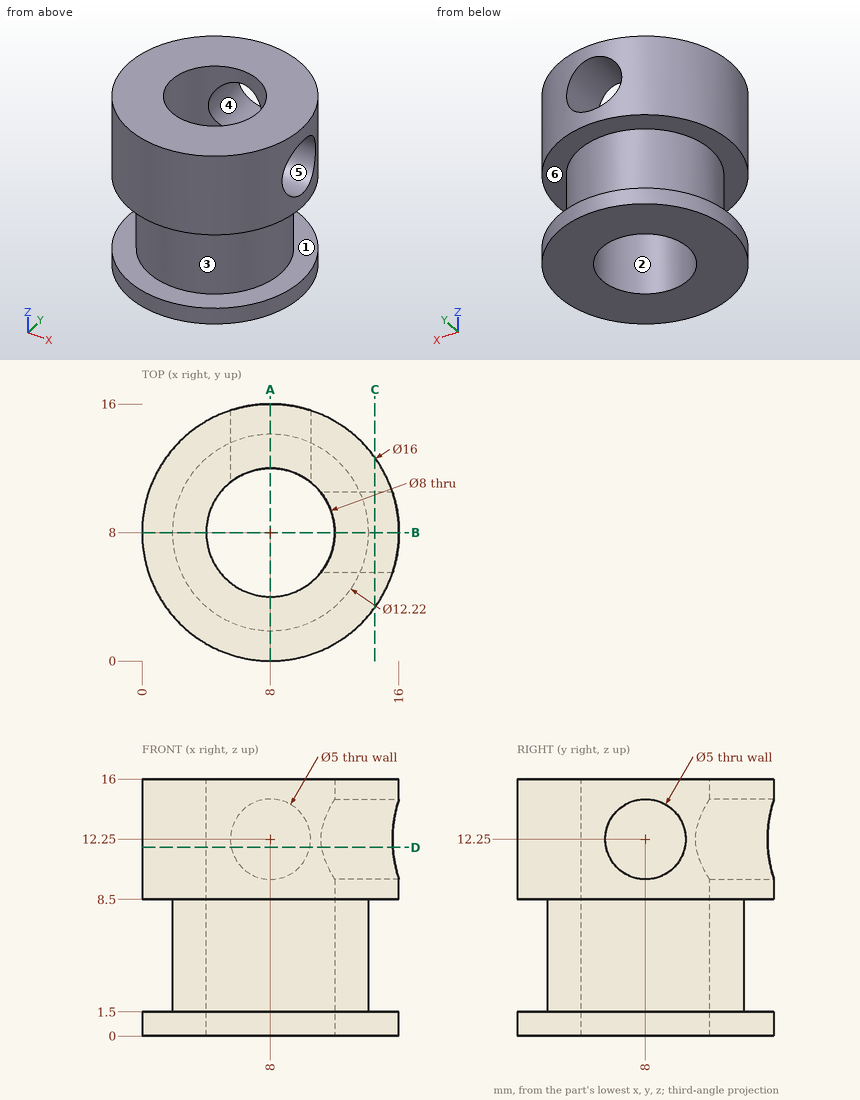
Job drawing, mm, ordinate dimensions from the low corner. One solid piece. A direction names the side the tool comes from. Coordinates: 2 decimals unless noted, no trailing zeros. Order: outer loops, then holes, each group sorted by start corner. A loop starts at its lowest first (then second) coordinate and runs counter-clockwise, first axis right, second up. Notation, with made-up numbers: (-4, 62) -> (46, 62) arc R19 cw to (46, 77) -> close; hole circle Ø7 at (12, 5.5). An arc over 180 degrees is marked (long way). Return JSON: item names as keys, results as strings. Group by question number.
Item 1: Saw through at A-A on x = 8. Write the cut outline in (y, z), then the cut area to 3 significant figures.
Item 2: Flat gauge pins, fed straight in: P1, Ø5, axis at x = 13.5, z = 9, coming from the -Y side; P2, Ø4, axis at y = 5.5, z = 13, coming from the +X side; P3, Ø4, axis at x = 5.5, z = 10.5, coming from the -Y side. Where does each tip first touch, or does it go through?
Item 3: Saw through at D-D on z = 11.75. Write the cut outline in (x, y), then the cut area to 3 significant figures.
Item 4: Saw through at C-C on x = 14.5. Write the cut outline in (y, z), then the cut area to 3 significant figures.
Item 5: Pull direction Y, two halves, no side cores. Call the marked faces 1, 2 and 3: pulls with the +Y half, pulls with the -Y half, needs draft (parallel to the pull), parting line crosses it, or undercut.
Item 6: Wall check: line 1 along Y through (x, z) = (8, 3.75); line 2 along X through (y, z) = (10.5, 4.5); line 3 along Z through (x, y) = (2.5, 13.75). Give the ranges that are in metal, low to high. Write a range as [from, to].
Item 7: Tool access for the marked faces 4, 5 and 6: list every direction of +Z, -Z, +X, -X, +Y, -Y with a clear straight run to the whole face (end or side of a thin tool).
Values found:
{
 "1": {"outline": "(0, 0) -> (4, 0) -> (4, 16) -> (0, 16) -> (0, 8.5) -> (1.89, 8.5) -> (1.89, 1.5) -> (0, 1.5) -> close; (12, 0) -> (16, 0) -> (16, 1.5) -> (14.11, 1.5) -> (14.11, 8.5) -> (16, 8.5) -> (16, 9.75) -> (12, 9.75) -> close; (12, 14.75) -> (16, 14.75) -> (16, 16) -> (12, 16) -> close", "area": "81.5 mm2"},
 "2": {"P1": "stops at y = 0.58", "P2": "stops at x = 15.92", "P3": "stops at y = 0.02"},
 "3": {"outline": "(5.55, 11.16) -> (5.55, 15.62) arc R8 ccw (long way) to (15.62, 5.55) -> (11.16, 5.55) arc R4 cw (long way) to start; (10.45, 11.16) arc R4 cw to (11.16, 10.45) -> (15.62, 10.45) arc R8 ccw to (10.45, 15.62) -> close", "area": "110 mm2"},
 "4": {"outline": "(3.34, 0) -> (12.66, 0) -> (12.66, 1.5) -> (3.34, 1.5) -> close; (3.34, 8.5) -> (12.66, 8.5) -> (12.66, 16) -> (3.34, 16) -> close; hole circle Ø5 at (8, 12.25)", "area": "64.3 mm2"},
 "5": {"face 1": "needs draft", "face 2": "undercut", "face 3": "parting line crosses it"},
 "6": {"line 1": "y = [1.89, 4], [12, 14.11]", "line 2": "x = [2.42, 4.88], [11.12, 13.58]", "line 3": "z = [0, 1.5], [8.5, 16]"},
 "7": {"face 4": "+Y", "face 5": "+X", "face 6": "none"}
}
